Answer from the drawing. Dimensions are ordinates in mm from the lowest x, y and z of the part. A direction names the side the tool comes from. Give positions to 0.01 mm unless a question says otherwise; leave off trailing zeros. Loops run counter-clockwise (first coordinate to the right, second up) from the corner with the lowest first, then second, coordinate; pieces in that order, holes last.
(1) Which of the six approach directions +Z, -Z, +X, -X, +Y, -Y give full straight-line access (tool end or side, diameter ignored) to the marked faces 1, 2 and 3?
(2) Each of these flat-tipped pins is pushed along its axis until it touches: P1, Ø8, axis at y = 6, z = 32, coming from the -X side; P2, Ø5, axis at y = 23.5, z = 14, coming from the +X side (1 decimal); P3, Ø12, axis at x = 78, y = 3, coming from the -Z side. Where does it stop, or does it pass through?
(3) Find section A-A, the plane y = 28. Write down the section's boundary in (x, z), then the cut area to 3 significant figures.
(4) Straight lines are drawn through the part: probe 1 along Y at (x, z) = (19.05, 10); probe 2 along Z at (x, y) = (34.5, 3); probe 3 along X at (y, z) = (14, 9) (1 decimal). For each, find the intervals that lie inside material, in ascending order.
(5) Determine the mould class of the marked faces 4, 5 and 6 for opening direction Y: pulls with the +Y half, pulls with the -Y half, needs draft (parallel to the pull), parting line crosses it, or undercut.
(6) Find section B-B, the plane x = 19.05. Write down the section's boundary in (y, z), then the cut area to 3 significant figures.
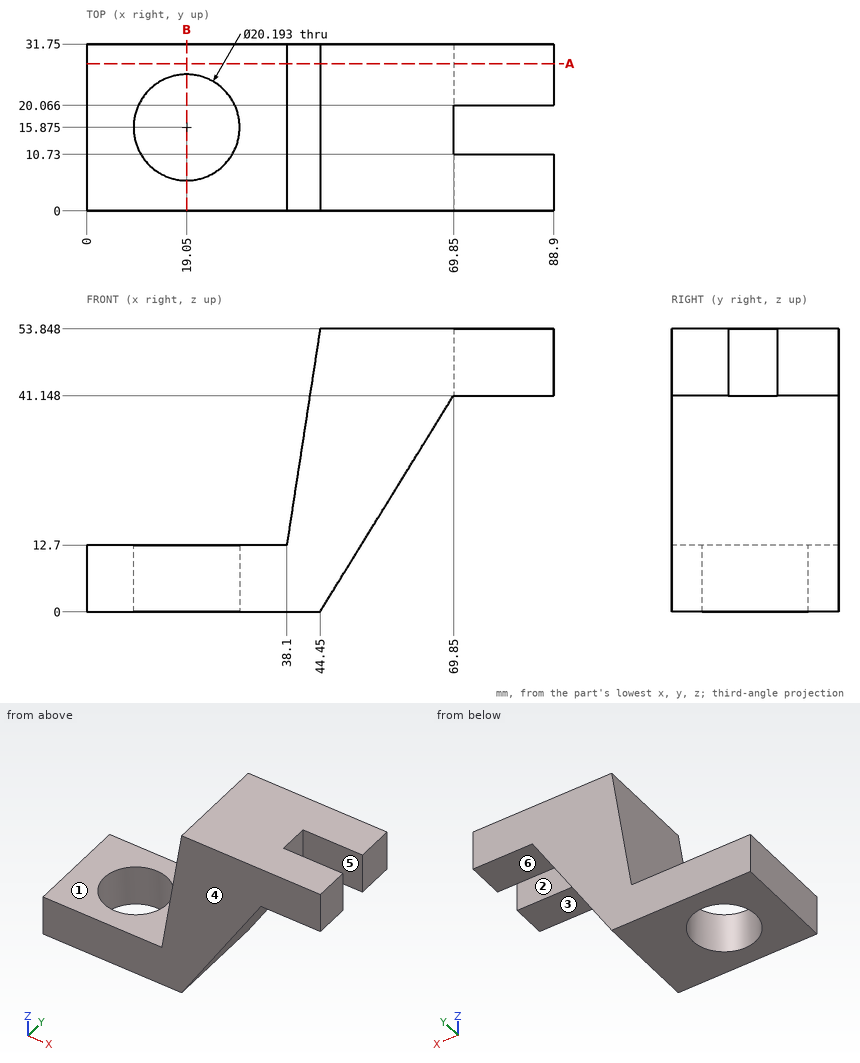
Entries:
1. face 1: +Z, -X, +Y, -Y
1. face 2: +Z, -Z, +X
1. face 3: -Z, +X, +Y, -Y
2. P1: stops at x = 40.46
2. P2: stops at x = 54.6
2. P3: stops at z = 41.15
3. outline: (0, 0) - (44.45, 0) - (69.85, 41.15) - (88.9, 41.15) - (88.9, 53.85) - (44.45, 53.85) - (38.1, 12.7) - (0, 12.7) - close
3. area: 1,780 mm2
4. probe 1: y = 0 to 5.78, 25.97 to 31.75
4. probe 2: z = 0 to 12.7
4. probe 3: x = 0 to 9.1, 29 to 50
5. face 4: pulls with the -Y half
5. face 5: undercut
5. face 6: needs draft
6. outline: (0, 0) - (5.78, 0) - (5.78, 12.7) - (0, 12.7) - close; (25.97, 0) - (31.75, 0) - (31.75, 12.7) - (25.97, 12.7) - close
6. area: 147 mm2
